The model under review builds one solid part; all positions refer to its coordinate system, in mm. A direction names the side the tool comes from. Coordinates: 2 decimals unless noted, no trailing zeros. Loops run counter-clockwise (first coordinate to the right, second up) from the corner with the lowest first, then second, coordinate; pieces in that order, holes last. Notation, with made-up numbers: (38.5, 76.5) - (61.5, 76.5) arc R22 cw to (61.5, 107.5) - close; hole circle Ø11 at (65.5, -7). An arc over 180 degrees is marked (long way). One line per item, written item: value. Start each with the question number.
1. Insertion check: P1, Ø3, axis at y = -2.5, z = 41, coming from the +X side; P2, Ø5, axis at x = -56, z = 8, coming from the +Y side; P3, Ø2.5, axis at x = 56, z = 8, coming from the +Y side; P4, Ø1.8, axis at x = -7, y = -3.5, coming from the -Z side. Each pin has a flat end and moves straight along its axis. Give the tip position at first contact, or say it passes through.
2. Mouldability with a two-part tool opening along Z and no side actions: class faces 5 (the face through (55, -3, 0)), 6 (the face through (49.5, -3, 25)), 7 (the face through (57.897, -4.176, 7.917)) as +Z half, -Z half, draft (parallel to the pull), parting line (faces both ways), or undercut.
3. We need section D-D, the plane z = 8. Give the boundary of the cut face in (x, y), then the cut area to 3 significant figures.
4. To check wall thickness, follow line 1 (X direction, y = -4.15, z = 8); line 2 (X direction, y = -2.95, z = 35); line 3 (Z direction, x = 56, y = -4.1). State the ranges of each line that lie inside material, in increasing order.
5. We need section C-C, the plane x = -56. Give the boundary of the cut face in (y, z), then the cut area to 3 significant figures.
6. We need section B-B, the plane y = -3.8. Give the boundary of the cut face in (x, z), then the cut area to 3 significant figures.
7. For faces 1 (the face through (61.5, -3, 25)), 2 (the face through (-50.5, -3, 25)), 3 (the face through (-75, -3, 50)), 4 (the face through (0, 0, 51)), list the 3-axis set-ups (+Z, -Z, +X, -X, +Y, -Y) from which the entire face can be reached by the end or side of a thin tool; tool diameter is ignored.
8. We need section A-A, the plane z = 35.5. Give the boundary of the cut face in (x, y), then the cut area to 3 significant figures.
from build123d import *

# Parameters (mm, degrees)
F1_DEPTH       = 6
F2_D           = 3.7973
F2_CSINK_D     = 7.7978
F2_CSINK_ANGLE = 82


with BuildPart() as f1:
    # F0 (on Front) → F1 (new body)
    with BuildSketch(Plane.XZ):
        Polygon((-87.5, 58), (-87.5, 50), (-62.5, 50), (-62.5, 0), (-50.5, 0), (-50.5, 50), (49.5, 50), (49.5, 0), (61.5, 0), (61.5, 50), (87.5, 50), (87.5, 58), align=None)
    extrude(amount=F1_DEPTH)

    # F2 (through all)
    with Locations(Plane(origin=(0, 0, 0), x_dir=(1, 0, 0), z_dir=(0, 1, 0))):
        with Locations((-56, -8), (56, -8)):
            CounterSinkHole(F2_D / 2, F2_CSINK_D / 2, counter_sink_angle=F2_CSINK_ANGLE)


solid = f1.part
Findings below:
1. P1: x = 61.5
1. P2: y = -1.61
1. P3: through
1. P4: z = 50
2. face 5: -Z half
2. face 6: draft
2. face 7: undercut
3. outline: (-62.5, -6) - (-57.9, -6) - (-57.9, -2.3) - (-59.9, 0) - (-62.5, 0) - close; (-54.1, -6) - (-50.5, -6) - (-50.5, 0) - (-52.1, 0) - (-54.1, -2.3) - close; (49.5, -6) - (54.1, -6) - (54.1, -2.3) - (52.1, 0) - (49.5, 0) - close; (57.9, -6) - (61.5, -6) - (61.5, 0) - (59.9, 0) - (57.9, -2.3) - close
3. area: 89.2 mm2
4. line 1: -62.5 to -57.9, -54.1 to -50.5, 49.5 to 54.1, 57.9 to 61.5
4. line 2: -62.5 to -50.5, 49.5 to 61.5
4. line 3: 0 to 6.1, 9.9 to 58
5. outline: (-6, 0) - (0, 0) - (0, 4.1) - (-2.3, 6.1) - (-6, 6.1) - close; (-6, 9.9) - (-2.3, 9.9) - (0, 11.9) - (0, 58) - (-6, 58) - close
5. area: 321 mm2
6. outline: (-87.5, 50) - (-62.5, 50) - (-62.5, 0) - (-50.5, 0) - (-50.5, 50) - (49.5, 50) - (49.5, 0) - (61.5, 0) - (61.5, 50) - (87.5, 50) - (87.5, 58) - (-87.5, 58) - close; hole circle Ø3.8 at (-56, 8); hole circle Ø3.8 at (56, 8)
6. area: 2,580 mm2
7. face 1: -Z, +X, +Y, -Y
7. face 2: -Z, +Y, -Y
7. face 3: -Z, -X, +Y, -Y
7. face 4: +Z, -Z, +X, -X, +Y
8. outline: (-62.5, -6) - (-50.5, -6) - (-50.5, 0) - (-62.5, 0) - close; (49.5, -6) - (61.5, -6) - (61.5, 0) - (49.5, 0) - close
8. area: 144 mm2
